```python
from build123d import *

# Parameters (mm, degrees)
SKETCH1_W           = 320
SKETCH1_H           = 200
BOSS_EXTRUDE1_DEPTH = 150
SHELL2_T            = 3


with BuildPart() as part:
    # Sketch1 → Boss-Extrude1 (new body)
    with BuildSketch(Plane(origin=(0, 0, 0), x_dir=(1, 0, 0), z_dir=(0, 1, 0))):
        with Locations((50.169491525, -5.762711864)):
            Rectangle(SKETCH1_W, SKETCH1_H)
    extrude(amount=BOSS_EXTRUDE1_DEPTH)

    # Shell2 (no face opened: a closed hollow body)
    add(offset(amount=-SHELL2_T, mode=Mode.PRIVATE), mode=Mode.SUBTRACT)


solid = part.part
```
Work out the finished part from the listing and answer in its coordinate system (mm). A direction names the side the tool comes from. Give positions to 0.01 mm unless a question says otherwise; leave off trailing zeros. Loops run counter-clockwise (first coordinate to the right, second up) from the corner with the lowest first, then second, coordinate; pieces in that order, holes last. Notation, with made-up numbers: M 7.5,28 L 38.5,28 A32 cw 38.5,57 Z; hole C 39,-6 d5. An arc over 180 degrees is marked long. One line per item, written item: value. Start each with the question number.
1. Find the intervals of material crossed by probe 1 along X at (y, z) = (56.5, 74); probe 2 along Z at (x, y) = (-20, 38); probe 3 along Y at (x, z) = (66.5, -2.5), in increasing order.
2. Which of the six approach directions +Z, -Z, +X, -X, +Y, -Y give full straight-line access (tool end or side, diameter ignored) to faces 5 (the face through (48, 74, -94.237)), 6 (the face through (48, 3, 4))?
3. Find section B-B (z = 32). Give the vertices of the cut face in (x, y), and give its area (3 significant figures).
4. Find section A-A (y = 60.5). Give the vertices of the cut face in (x, z).
5. Determine the mould class of faces 1 (the face through (48, 150, 4)), 2 (the face through (48, 74, -91.237)), 3 (the face through (-106.831, 74, 7)), 4 (the face through (-109.831, 74, 7)) for opening direction X: released by +X, released by -X, zero draft, split by the parting line, or undercut.
Reported:
1. probe 1: x = -109.83 to -106.83, 207.17 to 210.17
1. probe 2: z = -94.24 to -91.24, 102.76 to 105.76
1. probe 3: y = 0 to 3, 147 to 150
2. face 5: -Z, +X, -X, +Y, -Y
2. face 6: none
3. outline: M -109.83,0 L 210.17,0 L 210.17,150 L -109.83,150 Z; hole M -106.83,3 L 207.17,3 L 207.17,147 L -106.83,147 Z
3. area: 2,780 mm²
4. outline: M -109.83,-94.24 L 210.17,-94.24 L 210.17,105.76 L -109.83,105.76 Z; hole M -106.83,-91.24 L 207.17,-91.24 L 207.17,102.76 L -106.83,102.76 Z
5. face 1: zero draft
5. face 2: undercut
5. face 3: undercut
5. face 4: released by -X
